Read the model definition and answer for the solid it produces. Units are mm, in the model's axes. Face numbers are marked on the shaded views. Give positions to 0.01 mm unless a question says otherwise; leave off trailing zeros. Loops run counter-clockwise (first coordinate to the right, second up) from the corner with the lowest first, then second, coordinate; pieces in that order, holes last.
(1) Each of these flat-tipped pins is pushed along its axis until it touches: P1, Ø1.5, axis at x = -32, z = 113, coming from the +Y side; P2, Ø4, axis at x = 6.5, z = 288, coming from the -Y side; P3, Ø12, axis at x = 19, z = 347, coming from the -Y side. Where does it stop, or does it pass through?
(2) Determine the mould class of the marked faces 1 and 2 for opening direction Y: pulls with the +Y half, pulls with the -Y half, needs draft (parallel to the pull), parting line crosses it, or undercut.
(3) Find section C-C, the plane z = 233. Write down the section's boundary in (x, y).
(4) Find section A-A, the plane y = -26. Write down the section's boundary in (x, z).
(5) Find section B-B, the plane x = -15. Write down the section's boundary in (y, z), then the cut area to 3 significant figures.
(6) Straight lines are drawn through the part: probe 1 along Z at (x, y) = (0, 44); probe 2 along X at (y, z) = (5.5, 248.5); probe 3 along Y at (x, z) = (12, 329). For each, find the intervals that lie inside material, in ascending order.
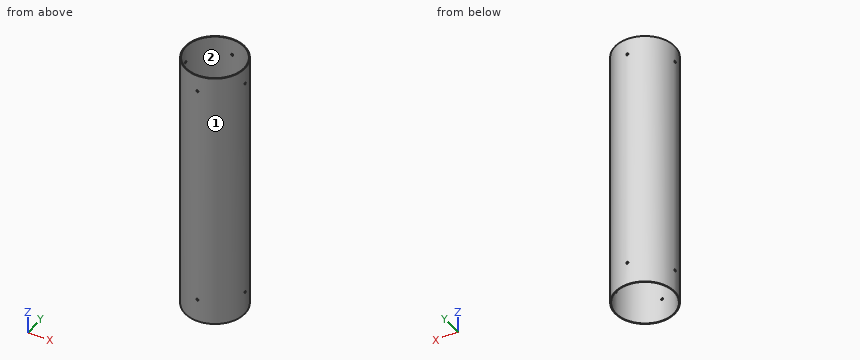
```python
from build123d import *

# Parameters (mm, degrees)
SKETCH1_R           = 45
SKETCH1_R_2         = 43.75
BOSS_EXTRUDE1_DEPTH = 400
SKETCH2_R           = 1.65
CUT_EXTRUDE1_DEPTH  = 406.030863022
CIRPATTERN1_COUNT   = 4


with BuildPart() as part:
    # Sketch1 → Boss-Extrude1 (new body)
    with BuildSketch(Plane.XY):
        Circle(SKETCH1_R)
        Circle(SKETCH1_R_2, mode=Mode.SUBTRACT)
    extrude(amount=BOSS_EXTRUDE1_DEPTH)

    # Sketch2 → Cut-Extrude1 (cut, through all)
    with BuildSketch(Plane(origin=(0, 0, 0), x_dir=(0, 0, -1), z_dir=(1, 0, 0))):
        with Locations((-35, 0)):
            Circle(SKETCH2_R)
        with Locations((-375, 0)):
            Circle(SKETCH2_R)
    cut_extrude1 = extrude(amount=-CUT_EXTRUDE1_DEPTH, mode=Mode.SUBTRACT)

    # CirPattern1: Cut-Extrude1 ×4 about axis
    cirpattern1_axis = Axis((0, 0, 400), (0, 0, -1))
    for i in range(1, CIRPATTERN1_COUNT):
        add(cut_extrude1.rotate(cirpattern1_axis, i * 360 / CIRPATTERN1_COUNT), mode=Mode.SUBTRACT)


solid = part.part
```
Entries:
1. P1: stops at y = 32.38
1. P2: stops at y = -44.77
1. P3: stops at y = -43.08
2. face 1: parting line crosses it
2. face 2: undercut
3. outline: circle Ø90 at (0, 0); hole circle Ø87.5 at (0, 0)
4. outline: (-36.73, 0) - (-35.19, 0) - (-35.19, 400) - (-36.73, 400) - close; (35.19, 0) - (36.73, 0) - (36.73, 400) - (35.19, 400) - close
5. outline: (-42.43, 0) - (-41.1, 0) - (-41.1, 400) - (-42.43, 400) - close; (41.1, 0) - (42.43, 0) - (42.43, 400) - (41.1, 400) - close
5. area: 1,060 mm2
6. probe 1: z = 0 to 33.35, 36.65 to 373.35, 376.65 to 400
6. probe 2: x = -44.66 to -43.4, 43.4 to 44.66
6. probe 3: y = -43.37 to -42.07, 42.07 to 43.37
